```python
from build123d import *

# Parameters (mm, degrees)
F0_W     = 127
F0_H     = 127
F1_DEPTH = 127
F3_D     = 19.05
F3_DEPTH = 12.7
F3_TIP   = 5.7231973962
F5_D     = 19.05
F5_DEPTH = 12.7
F5_TIP   = 5.7231973962


with BuildPart() as f1:
    # F0 (on Front) → F1 (new body)
    with BuildSketch(Plane.XZ):
        with Locations((-63.5, 63.5)):
            Rectangle(F0_W, F0_H)
    extrude(amount=F1_DEPTH)

    # F3
    with Locations(Plane.XZ.offset(127)):
        with Locations((-63.5, 101.6)):
            Hole(F3_D / 2, depth=F3_DEPTH)
            with Locations((0, 0, -(F3_DEPTH + F3_TIP / 2))):  # 118° drill point
                Cone(0, F3_D / 2, F3_TIP, mode=Mode.SUBTRACT)

    # F5
    with Locations(Plane.XY.offset(127)):
        with Locations((-63.5, -101.6)):
            Hole(F5_D / 2, depth=F5_DEPTH)
            with Locations((0, 0, -(F5_DEPTH + F5_TIP / 2))):  # 118° drill point
                Cone(0, F5_D / 2, F5_TIP, mode=Mode.SUBTRACT)


solid = f1.part
```
Input: part model. Units: mm. Frame: model coordinates. A direction names the side the tool comes from. Give positions to 0.01 mm unless a question says otherwise; leave off trailing zeros. One line per question, with ' | ' between items. Start each with the question number.
1. Pull-direction query (Y, two-part tool) for faces 3 (the face through (-62.7, -103.1, 109.6)), 4 (the face through (-64, 0, 64)), 5 (the face through (-72.585, -120.561, 104.461)), 6 (the face through (-62.61, -109.57, 102.99)); classes: released by +Y, released by -Y, zero draft, split by the parting line, or undercut.
2. Access query for faces 1 (the face through (-67.9, -110.05, 120.56)), 2 (the face through (-127, -63, 63)). Directions: +Z, -Z, +X, -X, +Y, -Y. A direction counts if a zero-diameter tool reaches every point of the face in a straight line with its end or side. Return the directions, or none.
3. Material intervals for probe 1 along Z at (x, y) = (-63.5, -119.25) (3 decimals); probe 2 along Y at (x, z) = (-63, 122); probe 3 along X at (y, z) = (-101.6, 123.75) (3 decimals), sorted ascending. Write a range as [from, to].
4. First-contact query: pin 1 Ø2 at (x, z) = (-102, 79) entering from +Y. Flat tip, straight axial feed; report the tip coordinate or a pass-through.
Here are the results:
1) face 3: undercut | face 4: released by +Y | face 5: zero draft | face 6: released by -Y
2) face 1: +Z | face 2: +Z, -Z, -X, +Y, -Y
3) probe 1: [0, 92.075], [111.125, 127] | probe 2: [-127, -111.11], [-92.09, 0] | probe 3: [-127, -73.025], [-53.975, 0]
4) pin 1: y = 0
